Job drawing, mm, ordinate dimensions from the low corner. One solid piece. A direction names the side the tool comes from. Give positions to 0.01 mm unless a question says otherwise; leave off trailing zeros. Loops run counter-clockwise (first coordinate to the right, second up) from the corner with the lowest first, then second, coordinate; pieces in that order, holes last.
Item 1: Saw through at D-D on z = 19.05. Give the cut face in (x, y), plus the area to 3 significant figures.
Item 2: Saw through at C-C on y = 10. Give the cut face in (x, z).
Item 3: Drop flat-ended pins along their axis: P1, Ø24, axis at x = 36.5, z = 25, coming from the +Y side; P2, Ø1.5, axis at x = 32.5, z = 20.5, coming from the +Y side; P3, Ø2, axis at y = 6, z = 34.5, coming from the +X side; P4, Ø2, axis at y = 7.5, z = 5, coming from the -X side. Give the stop position or say it passes through.
Item 4: Saw through at B-B on x = 35.95. Give the cut face in (y, z).
Item 5: Which spindle directions (+Z, -Z, +X, -X, +Y, -Y) get a long thin tool onto all of the face, cutting with end or side? Do the marked faces 4, 5 and 6. Say none if no direction does.
Item 6: Probe probe 1 along Z at (x, y) = (51.5, 3.3); probe 2 along Z at (x, y) = (51.5, 0.6); probe 3 along X at (y, z) = (2.65, 3.5). List the from-to ranges inside material, lowest first.
Item 7: Mould opens along Z. For the marked faces 1, 2 and 3 say: released by +Z, released by -Z, zero draft, split by the parting line, or undercut.
Item 8: Saw through at A-A on y = 1. Give the cut face in (x, z), plus the area to 3 significant figures.
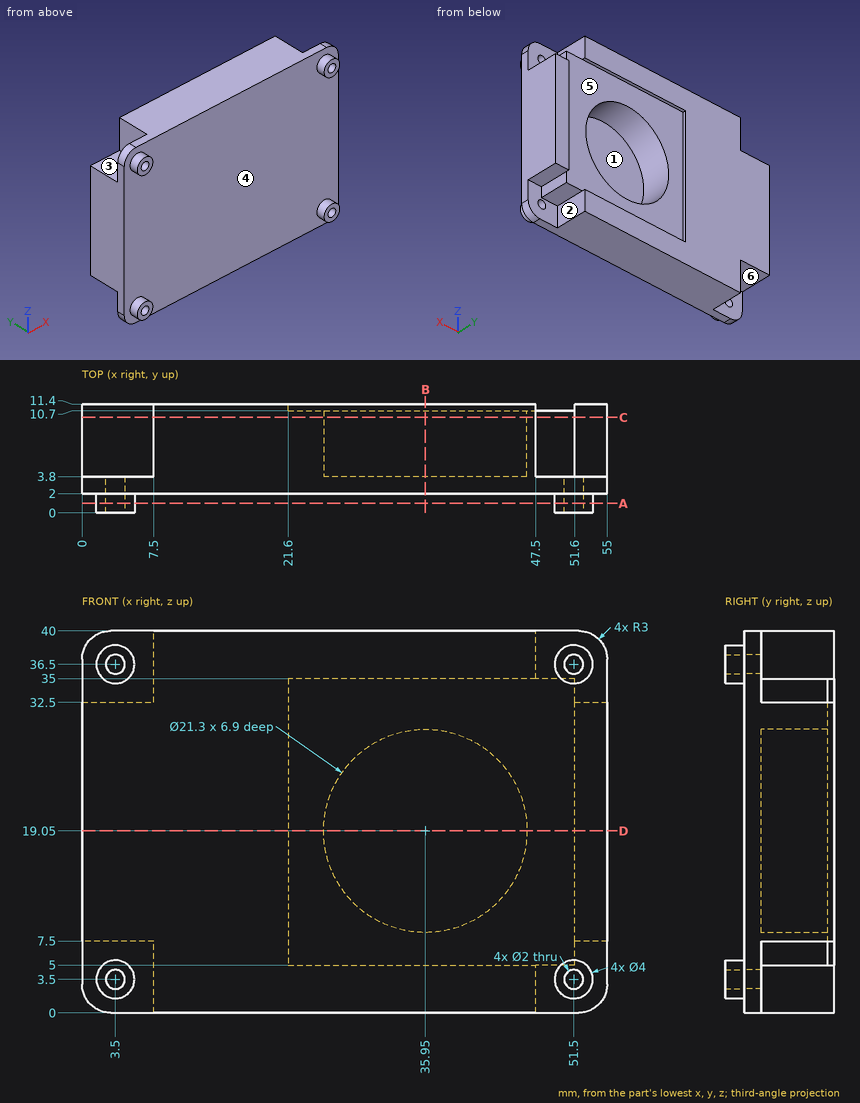
Results below:
1. outline: (0, 2) - (55, 2) - (55, 11.4) - (51.6, 11.4) - (51.6, 10.7) - (46.6, 10.7) - (46.6, 3.8) - (25.3, 3.8) - (25.3, 10.7) - (21.6, 10.7) - (21.6, 11.4) - (0, 11.4) - close
1. area: 349 mm2
2. outline: (0, 7.5) - (7.5, 7.5) - (7.5, 0) - (47.5, 0) - (47.5, 5) - (51.6, 5) - (51.6, 7.5) - (55, 7.5) - (55, 32.5) - (51.6, 32.5) - (51.6, 35) - (47.5, 35) - (47.5, 40) - (7.5, 40) - (7.5, 32.5) - (0, 32.5) - close; hole circle Ø21.3 at (35.95, 19.05)
3. P1: stops at y = 11.4
3. P2: stops at y = 3.8
3. P3: stops at x = 51.6
3. P4: stops at x = 7.5
4. outline: (2, 0) - (11.4, 0) - (11.4, 5) - (10.7, 5) - (10.7, 8.4) - (3.8, 8.4) - (3.8, 29.7) - (10.7, 29.7) - (10.7, 35) - (11.4, 35) - (11.4, 40) - (2, 40) - close
5. face 4: -Y
5. face 5: +Y
5. face 6: -Z, -X, +Y
6. probe 1: z = 0 to 2.5, 4.5 to 35.5, 37.5 to 40
6. probe 2: z = 1.5 to 2.5, 4.5 to 5.5, 34.5 to 35.5, 37.5 to 38.5
6. probe 3: x = 0 to 2.5, 4.5 to 50.5, 52.5 to 55
7. face 1: undercut
7. face 2: zero draft
7. face 3: released by +Z
8. outline: circle Ø4 at (3.5, 3.5); circle Ø4 at (3.5, 36.5); circle Ø4 at (51.5, 3.5); circle Ø4 at (51.5, 36.5); hole circle Ø2 at (3.5, 3.5); hole circle Ø2 at (3.5, 36.5); hole circle Ø2 at (51.5, 3.5); hole circle Ø2 at (51.5, 36.5)
8. area: 37.7 mm2
